from build123d import *

# Parameters (mm, degrees)
F0_W     = 381
F0_H     = 660.4
F0_W_2   = 355.6
F0_H_2   = 635
F1_DEPTH = 355.6
F2_DEPTH = 25.4
F3_W     = 76.2
F3_H     = 127
F4_DEPTH = 25.4
F5_W     = 127
F5_H     = 127
F6_DEPTH = 25.4


with BuildPart() as f1:
    # F0 (on Top) → F1 (new body)
    with BuildSketch(Plane.XY):
        Rectangle(F0_W, F0_H)
        Rectangle(F0_W_2, F0_H_2, mode=Mode.SUBTRACT)
    extrude(amount=F1_DEPTH)

    # F0 (on Top) → F2 (join)
    with BuildSketch(Plane.XY):
        Rectangle(F0_W_2, F0_H_2)
    extrude(amount=F2_DEPTH)

    # F3 (on face) → F4 (cut)
    with BuildSketch(Plane.XY):
        with Locations((-38.1, 143.031146)):
            Rectangle(F3_W, F3_H)
        with Locations((38.1, 143.031146)):
            Rectangle(F3_W, F3_H)
    extrude(amount=F4_DEPTH, mode=Mode.SUBTRACT)

    # F5 (on face) → F6 (cut)
    with BuildSketch(Plane(origin=(0, 330.2, 0), x_dir=(-1, 0, 0), z_dir=(0, 1, 0))):
        with Locations((0, 355.6)):
            Rectangle(F5_W, F5_H)
    extrude(amount=-F6_DEPTH, mode=Mode.SUBTRACT)


solid = f1.part
Geometry: final body of the model. Coordinates: model frame, mm. A direction names the side the tool comes from. Round coordinates to 2 decimals unless told otherwise and drop trailing zeros. Loops run counter-clockwise (first coordinate to the right, second up) from the corner with the lowest first, then second, coordinate; pieces in that order, holes last. Notation, with made-up numbers: (-23, 45.25) -> (-10, 45.25) arc R18 ccw to (-10, 59.25) -> close; hole circle Ø8 at (9, 1.25). An arc over 180 degrees is marked (long way). One line per question, with ' | ' between items. Start each with the question number.
1. Section D-D on y = 50. Output: boundary loops of the cut face in (x, z), and give its area (3 significant figures).
2. Section A-A on z = 227. Output: boundary loops of the cut face in (x, y), and give its area (3 significant figures).
3. Section C-C on z = 329. Output: boundary loops of the cut face in (x, y).
4. Line query: line 1 along X through (y, z) = (86.5, 317.5); line 2 along Y through (x, z) = (134, 71); line 3 along Z through (x, y) = (156.5, -280.5). Output: solid intervals per line, ascending. Write a range as [from, to].
5. Set-up query: faces 4 (the face through (1, 206.531, 13)), 5 (the face through (-2, -317.5, 188)), 6 (the face through (1, 324, 292.1)), 7 (the face through (-3, 5, 0)). Return all of +Z, -Z, +X, -X, +Y, -Y with unobstructed straight access to the full face (end or side cutting, diameter ignored); none if empty.
6. Section B-B on x = 45.5. Output: boundary loops of the cut face in (y, z).
7. Contact query for a flat-ended pin moving along its axis: pin 1 (6.5 mm diameter, centred on x = -19.5, y = 327, fed in from +Z). Output: stop coordinate, or through.
8. Mould query, pull axis X, two halves, no side actions, for faces 1 (the face through (-3, 330.2, 175)), 2 (the face through (63.5, 324, 323)), 3 (the face through (-190.5, -5, 175)). Classes: pulls with the +X half, pulls with the -X half, needs draft (parallel to the pull), parting line crosses it, or undercut.
Returned:
1) outline: (-190.5, 0) -> (190.5, 0) -> (190.5, 355.6) -> (177.8, 355.6) -> (177.8, 25.4) -> (-177.8, 25.4) -> (-177.8, 355.6) -> (-190.5, 355.6) -> close | area: 18,100 mm2
2) outline: (-190.5, -330.2) -> (190.5, -330.2) -> (190.5, 330.2) -> (-190.5, 330.2) -> close; hole (-177.8, -317.5) -> (177.8, -317.5) -> (177.8, 317.5) -> (-177.8, 317.5) -> close | area: 25,800 mm2
3) outline: (-190.5, -330.2) -> (190.5, -330.2) -> (190.5, 330.2) -> (63.5, 330.2) -> (63.5, 317.5) -> (177.8, 317.5) -> (177.8, -317.5) -> (-177.8, -317.5) -> (-177.8, 317.5) -> (-63.5, 317.5) -> (-63.5, 330.2) -> (-190.5, 330.2) -> close
4) line 1: x = [-190.5, -177.8], [177.8, 190.5] | line 2: y = [-330.2, -317.5], [317.5, 330.2] | line 3: z = [0, 25.4]
5) face 4: +Z, -Z | face 5: +Z | face 6: +Z, +Y | face 7: -Z, +X, -X, +Y, -Y
6) outline: (-330.2, 0) -> (79.53, 0) -> (79.53, 25.4) -> (-317.5, 25.4) -> (-317.5, 355.6) -> (-330.2, 355.6) -> close; (206.53, 0) -> (330.2, 0) -> (330.2, 292.1) -> (317.5, 292.1) -> (317.5, 25.4) -> (206.53, 25.4) -> close
7) pin 1: stops at z = 292.1
8) face 1: needs draft | face 2: undercut | face 3: pulls with the -X half
